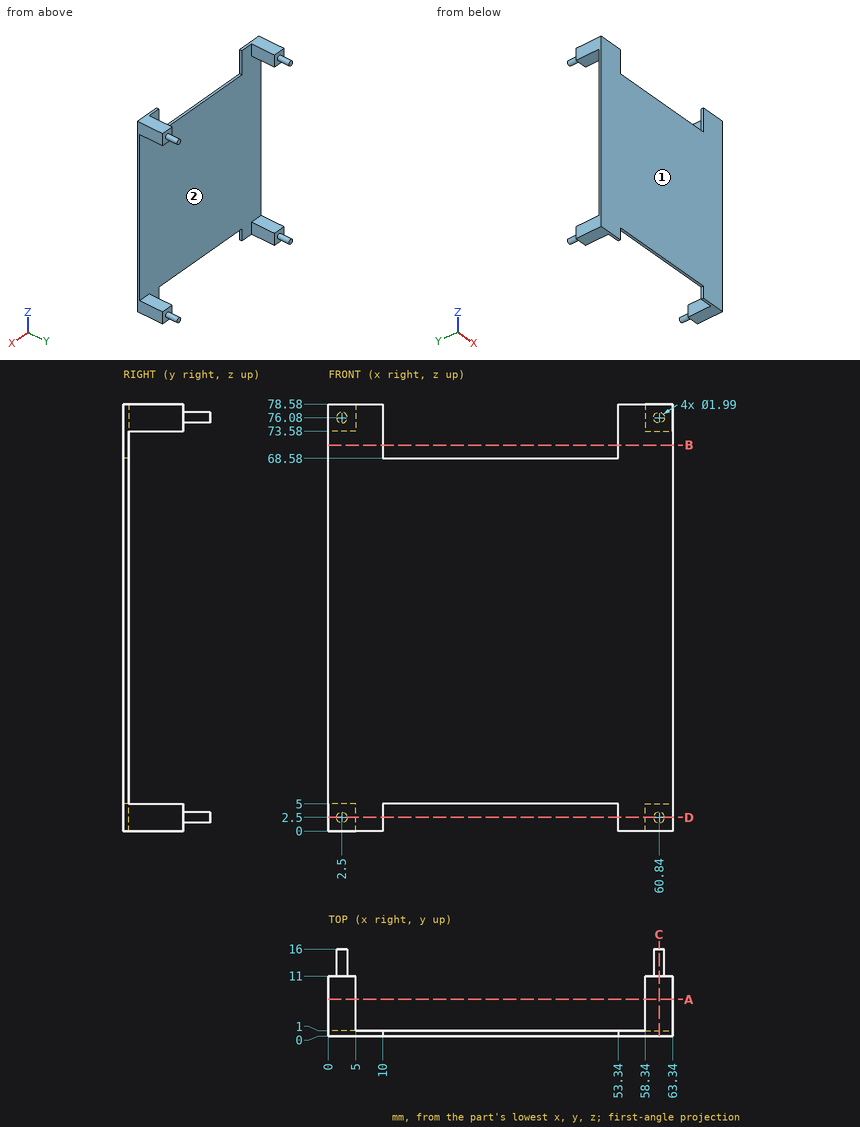
Design review of the part shown in the three views and the two pictorial views. Dimensions are in mm from the part's minimum x, y and z. Give positions to 0.01 mm unless a question says otherwise; leave off trailing zeros. Order: outer loops, then holes, each group sorted by start corner. A loop starts at its lowest first (then second) coordinate and runs counter-clockwise, first axis right, second up. Notation, with made-up numbers: (66, 52.5) -> (87, 52.5) arc R33 cw to (87, 83.5) -> close; hole circle Ø5 at (29.5, 1). An arc over 180 degrees is marked (long way). Write each question's results on one line, items separated by ' | '. Start each with the question number.
Q1. Add section A-A on y = 6.75. Give the boundary of the cut face in (x, z).
Q2. Add section D-D on z = 2.5. Give the boundary of the cut face in (x, y) (3 decimals).
Q3. For pin 1 (5 mm diameter, centred on y = 2.5, z = 66.5, fed in from +X); pin 2 (0.5 mm diameter, centred on x = 35, y = 0.5, fed in from +Z); pin 3 (6 mm diameter, centred on y = 5, z = 39, fed in from -X), all flat-tipped, find the tip position at first contact; note any pin that passes through.
Q4. Add section B-B on z = 71. Give the boundary of the cut face in (x, y).
Q5. Add section C-C on x = 60.84. Give the boundary of the cut face in (y, z) (3 decimals).
Q6. Wall thickness on L1, parallel to Z at x = 3.5, y = 9; L2, parallel to Y at x = 11.5, z = 63.5; L3, parallel to Z at x = 3, y = 13.25: over which ranges is each line inside the solid? List them lowest first. Write a range as from..to.
Q7. Mouldability with a two-part tool opening along Z and no side actions: class the marked faces 1 and 2 as +Z half, -Z half, draft (parallel to the pull), parting line (faces both ways), or undercut.
Found:
1) outline: (0, 0) -> (5, 0) -> (5, 5) -> (0, 5) -> close; (0, 73.58) -> (5, 73.58) -> (5, 78.58) -> (0, 78.58) -> close; (58.34, 0) -> (63.34, 0) -> (63.34, 5) -> (58.34, 5) -> close; (58.34, 73.58) -> (63.34, 73.58) -> (63.34, 78.58) -> (58.34, 78.58) -> close
2) outline: (0, 0) -> (10, 0) -> (10, 1) -> (5, 1) -> (5, 11) -> (3.495, 11) -> (3.495, 16) -> (1.505, 16) -> (1.505, 11) -> (0, 11) -> close; (53.34, 0) -> (63.34, 0) -> (63.34, 11) -> (61.835, 11) -> (61.835, 16) -> (59.845, 16) -> (59.845, 11) -> (58.34, 11) -> (58.34, 1) -> (53.34, 1) -> close
3) pin 1: stops at x = 63.34 | pin 2: stops at z = 68.58 | pin 3: passes through
4) outline: (0, 0) -> (10, 0) -> (10, 1) -> (0, 1) -> close; (53.34, 0) -> (63.34, 0) -> (63.34, 1) -> (53.34, 1) -> close
5) outline: (0, 0) -> (11, 0) -> (11, 1.505) -> (16, 1.505) -> (16, 3.495) -> (11, 3.495) -> (11, 5) -> (1, 5) -> (1, 73.58) -> (11, 73.58) -> (11, 75.085) -> (16, 75.085) -> (16, 77.075) -> (11, 77.075) -> (11, 78.58) -> (0, 78.58) -> close
6) L1: z = 0..5, 73.58..78.58 | L2: y = 0..1 | L3: z = 1.64..3.36, 75.22..76.94
7) face 1: draft | face 2: undercut
